Input: part model. Units: mm. Frame: model coordinates. Give positions to 0.01 mm unless a question says otherwise; leave off trailing zeros. Loops run counter-clockwise (first coordinate to the right, second up) from the corner with the lowest first, then second, coordinate; pieces in that order, holes last. Notation, with made-up numbers: M 78,20.25 L 110,20.25 A12 ccw 110,32.25 Z; hole C 18,73 d8. An arc over 180 degrees is marked long. Use CSV: the item, a comma, the result in double quotes. Start each with the question number.
Q1. Material intervals for line 1 along Z through (x, y) = (0, -15); line 2 along X through (y, z) = (-8, 0.95); line 3 along Y through (x, z) = (-1, 2.25), sorted ascending.
Q2. Section A-A, the plane y = -52.5. Output: boundary loops of the cut face in (x, z), plus the area to 3 significant figures.
Q3. Section B-B, the plane z = 1.5. Output: boundary loops of the cut face in (x, y).
Q4. Pin query (flat end, axial travel): pin 1 (3 mm diameter, centred on x = 0.5, y = -15, fed in from -Z); pin 2 (1 mm diameter, centred on x = -0.5, z = 1.5, fed in from +Y); pin 3 (1 mm diameter, centred on x = -3, z = 1.5, fed in from -Y). Return the tip coordinate at first contact, or that it passes through.
Q5. Section C-C, the plane x = 0.5. Output: boundary loops of the cut face in (y, z).
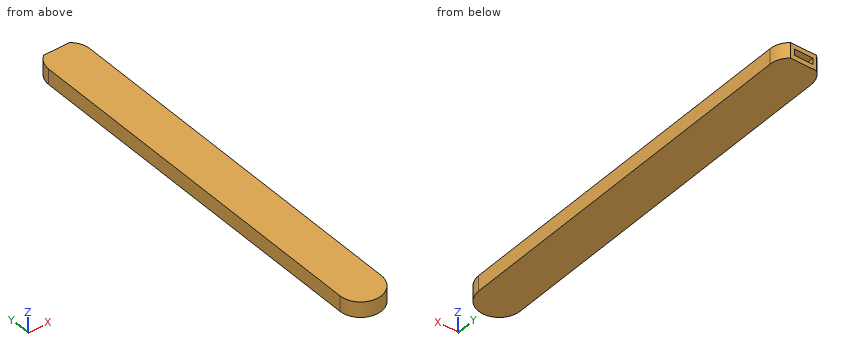
from build123d import *

# Parameters (mm, degrees)
F1_DEPTH = 3
F2_W     = 3.6
F2_H     = 1.2
F3_DEPTH = 60


with BuildPart() as f1:
    # F0 (on Top) → F1 (new body)
    with BuildSketch(Plane.XY):
        with BuildLine():
            Line((4.021343, -70.877558), (4.021343, 0))
            ThreePointArc((4.021343, 0), (3.626894, 1.732051), (2.521343, 3.122499))
            Line((2.521343, 3.122499), (-2.478657, 3.122499))
            ThreePointArc((-2.478657, 3.122499), (-3.584208, 1.732051), (-3.978657, 0))
            Line((-3.978657, 0), (-3.978657, -70.877558))
            ThreePointArc((-3.978657, -70.877558), (0.021343, -74.877558), (4.021343, -70.877558))
        make_face()
    extrude(amount=F1_DEPTH)

    # F2 (on face) → F3 (cut)
    with BuildSketch(Plane(origin=(0, 3.122499, 0), x_dir=(-1, 0, 0), z_dir=(0, 1, 0))):
        with Locations((0, 1.5)):
            Rectangle(F2_W, F2_H)
    extrude(amount=-F3_DEPTH, mode=Mode.SUBTRACT)


solid = f1.part
A:
1,line 1,"0 to 0.9, 2.1 to 3"
1,line 2,"-3.98 to -1.8, 1.8 to 4.02"
1,line 3,"-74.74 to 3.12"
2,outline,"M -3.98,0 L 4.02,0 L 4.02,3 L -3.98,3 Z; hole M -1.8,0.9 L 1.8,0.9 L 1.8,2.1 L -1.8,2.1 Z"
2,area,"19.7 mm^2"
3,outline,"M -3.98,-70.88 A4 ccw 4.02,-70.88 L 4.02,0 A4 ccw 2.52,3.12 L 1.8,3.12 L 1.8,-56.88 L -1.8,-56.88 L -1.8,3.12 L -2.48,3.12 A4 ccw -3.98,0 Z"
4,pin 1,"z = 0"
4,pin 2,"y = -56.88"
4,pin 3,"y = -73.98"
5,outline,"M -74.85,0 L 3.12,0 L 3.12,0.9 L -56.88,0.9 L -56.88,2.1 L 3.12,2.1 L 3.12,3 L -74.85,3 Z"
